Autodesk Inventor part; units mm, degrees
ref_plane "YZ Plane" through (0, 0, 0) normal (1, 0, 0) x (0, 1, 0)
ref_plane "XZ Plane" through (0, 0, 0) normal (0, 1, 0) x (-1, 0, 0)
ref_plane "XY Plane" through (0, 0, 0) normal (0, 0, 1) x (1, 0, 0)
sketch "Sketch1" plane through (0, 0, 0) normal (0, 0, 1) x (1, 0, 0)
  line L0 (15, 0) -> (15, 13)
  line L1 (0, 13) -> (0, 0)
  arc A0 (15, 13) -> (0, 13) centre (7.5, 13) ccw
  circle A1 centre (7.5, 13) radius 2.5
  line L2 (0, 0) -> (3, 0)
  line L3 (3, 0) -> (3, 3)
  line L4 (0, 3) -> (0, 0)
  line L5 (15, 0) -> (12, 0)
  line L6 (12, 0) -> (12, 3)
  line L7 (15, 3) -> (15, 0)
  line L8 (3, 3) -> (12, 3)
  line L9 (0, 0) -> (3, 0)
  line L10 (12, 0) -> (15, 0)
  dimension "d0" = 15
  dimension "d1" = 13
  dimension "d2" = 5
extrude "Extrusion1" add sketch "Sketch1" along normal blind 3
properties part number "Connector_2"
Geometry: final body of the model. Coordinates: model frame, mm. A direction names the side the tool comes from. Round coordinates to 2 decimals unless told otherwise and drop trailing zeros. Loops run counter-clockwise (first coordinate to the right, second up) from the corner with the lowest first, then second, coordinate; pieces in that order, holes last. Notation, with made-up numbers: (74, 7) -> (106, 7) arc R26 cw to (106, 37) -> close; hole circle Ø2 at (74.25, -20.5). An arc over 180 degrees is marked (long way). One line per question, with ' | ' between items. Start each with the question number.
1. Mould query, pull axis X, two halves, no side actions, for faces 1 (the face through (7.34, 20.5, 1.48)), 2 (the face through (15, 6, 1)), 3 (the face through (7, 3, 1)). Classes: pulls with the +X half, pulls with the -X half, needs draft (parallel to the pull), parting line crosses it, or undercut.
2. Set-up query: faces 4 (the face through (1, 0, 1)), 5 (the face through (12, 1, 1)). Return all of +Z, -Z, +X, -X, +Y, -Y with unobstructed straight access to the full face (end or side cutting, diameter ignored); none if empty.
3. Line query: line 1 along Y through (x, z) = (7.5, 1.25); line 2 along Y through (x, z) = (5.75, 0.3); line 3 along X through (y, z) = (13.75, 0.6). Output: solid intervals per line, ascending. Write a range as [from, to].
4. Section C-C on y = 11. Output: boundary loops of the cut face in (x, z), and give its area (3 significant figures).
5. Section B-B on z = 1.6. Output: boundary loops of the cut face in (x, y).
6. Section D-D on y = 18.25. Output: boundary loops of the cut face in (x, z), and give its area (3 significant figures).
7. Section A-A on x = 7.5. Output: boundary loops of the cut face in (y, z).
8. Contact query for flat-ended pins moving along their axis: pin 1 (1 mm diameter, centred on x = 12, y = 10, fed in from -Z); pin 2 (1.5 mm diameter, centred on x = 5.5, z = 1, fed in from -Y). Output: stop coordinate, or through.
Returned:
1) face 1: parting line crosses it | face 2: pulls with the +X half | face 3: undercut
2) face 4: +Z, -Z, +X, -X, -Y | face 5: +Z, -Z, -Y
3) line 1: y = [3, 10.5], [15.5, 20.5] | line 2: y = [3, 11.21], [14.79, 20.29] | line 3: x = [0.04, 5.12], [9.88, 14.96]
4) outline: (0, 0) -> (6, 0) -> (6, 3) -> (0, 3) -> close; (9, 0) -> (15, 0) -> (15, 3) -> (9, 3) -> close | area: 36.0 mm2
5) outline: (0, 0) -> (3, 0) -> (3, 3) -> (12, 3) -> (12, 0) -> (15, 0) -> (15, 13) arc R7.5 ccw to (0, 13) -> close; hole circle Ø5 at (7.5, 13)
6) outline: (2.14, 0) -> (12.86, 0) -> (12.86, 3) -> (2.14, 3) -> close | area: 32.1 mm2
7) outline: (3, 0) -> (10.5, 0) -> (10.5, 3) -> (3, 3) -> close; (15.5, 0) -> (20.5, 0) -> (20.5, 3) -> (15.5, 3) -> close
8) pin 1: stops at z = 0 | pin 2: stops at y = 3
